Print and shaded views of the part. All mm, measured from the part's lowest x, y and z. Round coordinates to 2 decimals unless told otherwise and drop trailing zeros. Order: outer loops, then holes, each group sorted by start corner. A loop starts at its lowest first (then second) coordinate and runs counter-clockwise, first axis right, second up. Notation, with made-up numbers: (-1, 77) -> (29, 77) arc R11 ccw to (29, 91) -> close; hole circle Ø6 at (29.5, -5). An arc over 180 degrees is marked (long way). Answer as CSV lines item,"result". Start each with the question number.
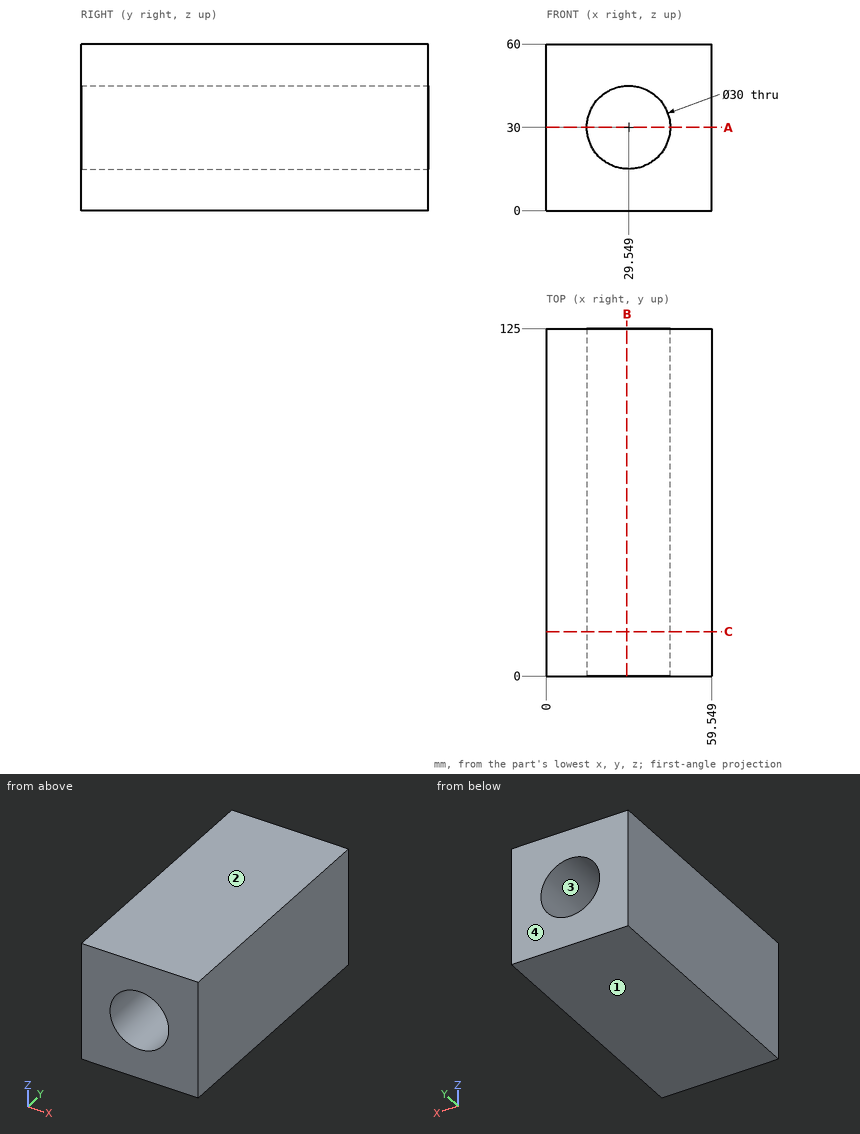
Item 1: Probe line 1 (Z direction, x = 29.5, y = 76.5); line 2 (Z direction, x = 27, y = 109); line 3 (X direction, y = 94.5, z = 32) (1 decimal). List the from-to ranges inside material, lowest first.
Item 2: Band-saw the part on B-B, the plane x = 29. Give the cut face in (y, z), and give its area (3 significant figures).
Item 3: Mould opens along Z. For the marked faces 1, 2, 3 and 4 say: released by +Z, released by -Z, zero draft, split by the parting line, or undercut.
Item 4: Band-saw the part on A-A, the plane z = 30. Give the cut face in (x, y).
Item 5: Band-saw the part on C-C, the plane y = 16. Give the cut face in (x, z), and give its area (3 significant figures).
Values:
1,line 1,"0 to 15, 45 to 60"
1,line 2,"0 to 15.22, 44.78 to 60"
1,line 3,"0 to 14.7, 44.4 to 59.5"
2,outline,"(0, 0) -> (125, 0) -> (125, 15.01) -> (0, 15.01) -> close; (0, 44.99) -> (125, 44.99) -> (125, 60) -> (0, 60) -> close"
2,area,"3,750 mm²"
3,face 1,"released by -Z"
3,face 2,"released by +Z"
3,face 3,"undercut"
3,face 4,"zero draft"
4,outline,"(0, 0) -> (14.55, 0) -> (14.55, 125) -> (0, 125) -> close; (44.55, 0) -> (59.55, 0) -> (59.55, 125) -> (44.55, 125) -> close"
5,outline,"(0, 0) -> (59.55, 0) -> (59.55, 60) -> (0, 60) -> close; hole circle Ø30 at (29.55, 30)"
5,area,"2,870 mm²"
